```python
from build123d import *

# Parameters (mm, degrees)
SKETCH_1_R          = 12.65
SKETCH_1_R_2        = 5.875
EXTRUDE_1_DEPTH     = 2
SKETCH_2_R          = 9.5
SKETCH_2_R_2        = 5
EXTRUDE_2_DEPTH     = 20
CHAMFER_1_SIZE      = 0.5
SKETCH_3_R          = 12.65
SKETCH_3_R_2        = 9.5
EXTRUDE_3_DEPTH     = 1.8
CHAMFER_2_SIZE      = 1
CHAMFER_4_SIZE      = 0.5
SKETCH_4_R          = 5
SKETCH_4_R_2        = 3
EXTRUDE_4_DEPTH     = 2
SKETCH_7_R          = 5.9
CUT_EXTRUDE_1_DEPTH = 0.3
CHAMFER_5_SIZE      = 0.5
SKETCH_8_R          = 3.25
CUT_EXTRUDE_2_DEPTH = 0.6
CHAMFER_6_SIZE      = 0.5


with BuildPart() as part:
    # 스케치1 → 보스-돌출1 (new body)
    with BuildSketch(Plane.XY):
        Circle(SKETCH_1_R)
        Circle(SKETCH_1_R_2, mode=Mode.SUBTRACT)
    extrude(amount=EXTRUDE_1_DEPTH)

    # 스케치2 → 보스-돌출2 (add)
    with BuildSketch(Plane.XY.offset(2)):
        Circle(SKETCH_2_R)
        Circle(SKETCH_2_R_2, mode=Mode.SUBTRACT)
    extrude(amount=EXTRUDE_2_DEPTH)

    # 모따기1
    chamfer_1_edges = [part.edges().sort_by_distance(p)[0] for p in [
        (-5.875, 0, 0),
    ]]
    chamfer(chamfer_1_edges, length=CHAMFER_1_SIZE)

    # 스케치3 → 보스-돌출3 (add)
    with BuildSketch(Plane.XY.offset(2)):
        Circle(SKETCH_3_R)
        Circle(SKETCH_3_R_2, mode=Mode.SUBTRACT)
    extrude(amount=EXTRUDE_3_DEPTH)

    # 모따기2
    chamfer_2_edges = [part.edges().sort_by_distance(p)[0] for p in [
        (-9.5, 0, 22),
    ]]
    chamfer(chamfer_2_edges, length=CHAMFER_2_SIZE)

    # 모따기4
    chamfer_4_edges = [part.edges().sort_by_distance(p)[0] for p in [
        (-12.65, 0, 0),
    ]]
    chamfer(chamfer_4_edges, length=CHAMFER_4_SIZE)

    # 스케치4 → 보스-돌출4 (add)
    with BuildSketch(Plane(origin=(0, 0, 2), x_dir=(-1, 0, 0), z_dir=(0, 0, -1))):
        Circle(SKETCH_4_R)
        Circle(SKETCH_4_R_2, mode=Mode.SUBTRACT)
    extrude(amount=-EXTRUDE_4_DEPTH)

    # 스케치7 → 컷-돌출1 (cut)
    with BuildSketch(Plane(origin=(0, 0, 2), x_dir=(-1, 0, 0), z_dir=(0, 0, -1))):
        Circle(SKETCH_7_R)
    extrude(amount=-CUT_EXTRUDE_1_DEPTH, mode=Mode.SUBTRACT)

    # 모따기5
    chamfer_5_edges = [part.edges().sort_by_distance(p)[0] for p in [
        (3, 0, 2.3),
    ]]
    chamfer(chamfer_5_edges, length=CHAMFER_5_SIZE)

    # 스케치8 → 컷-돌출2 (cut)
    with BuildSketch(Plane.XY.offset(4)):
        Circle(SKETCH_8_R)
    extrude(amount=-CUT_EXTRUDE_2_DEPTH, mode=Mode.SUBTRACT)

    # 모따기6
    # the kernel refuses this chamfer: 0.5 mm, written as the material it adds along each edge
    with BuildSketch(Plane(origin=(0, 0, 3.4), x_dir=(1, 0, 0), z_dir=(0, -1, 0))) as chamfer_6_piece_1_section:
        Polygon((3.25 - CHAMFER_6_SIZE, 0), (3.25, CHAMFER_6_SIZE), (3.25, 0), align=None)
    chamfer_6_piece_1 = revolve(axis=Axis((0, 0, 3.4), (0, 0, 1)), mode=Mode.PRIVATE)
    chamfer_6_piece_1 = chamfer_6_piece_1 - Plane(origin=(0, 0, 3.773130842), x_dir=(-1, 0, 0), z_dir=(0, 0, -1)) * Cylinder(3, 13, mode=Mode.PRIVATE)
    add(chamfer_6_piece_1)


solid = part.part
```
Verification items for the finished model (mm, model axes). A direction names the side the tool comes from. Round coordinates to 2 decimals unless told otherwise and drop trailing zeros. Write each loop counter-clockwise with the first axis right and the second up, starting at its lowest first coordinate (ties: lowest second). Pieces come first, ordered by that corner, then holes. Notation, with made-up numbers: (87.5, 15.5) -> (96.5, 15.5) arc R6 ccw to (96.5, 22.5) -> close; hole circle Ø2 at (-31, 87.5). An arc over 180 degrees is marked (long way). Write each question's results on one line, items separated by ' | '.
Q1. Draft check along X on faces 1 (the face through (4.38, -8.43, 12.28)), 2 (the face through (4, -4, 22)), 3 (the face through (3, 0, 3)). Enter one of: released by +X, released by -X, zero draft, split by the parting line, or undercut.
Derived:
face 1: split by the parting line | face 2: zero draft | face 3: undercut
Q2. Go/stop test with flat-tipped pins: pin 1 Ø2 at (x, y) = (-4.5, 1.5) entering from +Z; pin 2 Ø8 at (y, z) = (2, 10.5) entering from +X; pin 3 Ø6 at (x, y) = (0, 1.5) entering from +Z; pin 4 Ø10 at (y, z) = (-8, 9.5) entering from -X. Record where each tip stops, or that it passes through.
Derived:
pin 1: stops at z = 22 | pin 2: stops at x = 9.5 | pin 3: stops at z = 4 | pin 4: stops at x = -9.01
Q3. Thickness scan on probe 1 along Y at (x, z) = (0, 3.95); probe 2 along Y at (x, z) = (0, 3.1); probe 3 along Z at (x, y) = (5, 0.75). Record the ranges inside material, lowest first.
Derived:
probe 1: y = -9.5 to -3.25, 3.25 to 9.5 | probe 2: y = -12.65 to -3, 3 to 12.65 | probe 3: z = 2.3 to 22
Q4. Sectioned sample at A-A, the plane z = 6. Record the boundary of the cut face in (x, y).
Derived:
outline: circle Ø19 at (0, 0); hole circle Ø10 at (0, 0)
Q5. Access from +Z, -Z, +X, -X, +Y, -Y to the whole of each face (thin tool, end or side, straight path). Record for faces 4 (the face through (5.604, 1.765, 1.24)), 5 (the face through (-1.08, -4.88, 12.87)), 6 (the face through (5, -5, 0)).
Derived:
face 4: -Z | face 5: +Z | face 6: -Z, +X, -X, +Y, -Y
